Job drawing, mm, ordinate dimensions from the low corner. One solid piece. Give positions to 0.01 mm unless a question says otherwise; leave off trailing zeros. Loops run counter-clockwise (first coordinate to the right, second up) from the corner with the lowest first, then second, coordinate; pieces in that order, holes last.
Item 1: Saw through at C-C on z = 19. Give the cut face in (x, y).
Item 2: Saw through at A-A on z = 39.5. Give the cut face in (x, y) (1 decimal).
Item 3: Saw through at B-B on x = 20.5. Give the cut face in (y, z).
Item 4: Probe probe 1 along Z at (x, y) = (47, 1.85); probe 2 along X at (y, z) = (1.5, 20.5). List the from-to ranges inside material, lowest first.
Item 5: Drop flat-ended pins along their axis: P1, Ø0.9, axis at y = 2, z = 1, coming from the +X side (1 decimal); P2, Ø0.9, axis at y = 1.5, z = 36, coming from the +X side; P3, Ø0.9, axis at x = 1.5, y = 2, coming from the +Z side. Give the stop position or say it passes through.
Item 6: Saw through at D-D on y = 2.2. Give the number of separate pieces and of enclosed holes in the cut face, plus the area to 3 significant figures.
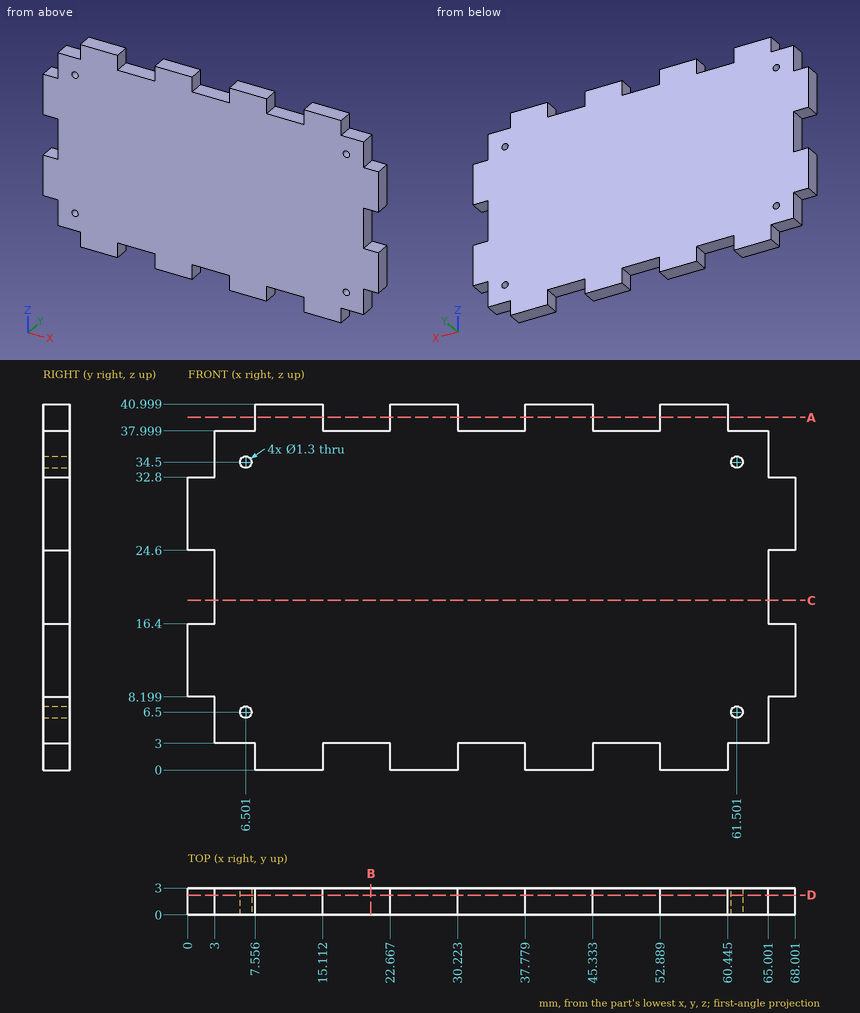
Results below:
1. outline: (3, 0) - (65, 0) - (65, 3) - (3, 3) - close
2. outline: (7.6, 0) - (15.1, 0) - (15.1, 3) - (7.6, 3) - close; (22.7, 0) - (30.2, 0) - (30.2, 3) - (22.7, 3) - close; (37.8, 0) - (45.3, 0) - (45.3, 3) - (37.8, 3) - close; (52.9, 0) - (60.4, 0) - (60.4, 3) - (52.9, 3) - close
3. outline: (0, 3) - (3, 3) - (3, 38) - (0, 38) - close
4. probe 1: z = 3 to 38
4. probe 2: x = 3 to 65
5. P1: stops at x = 60.4
5. P2: stops at x = 65
5. P3: stops at z = 32.8
6. separate pieces: 1
6. enclosed holes: 4
6. area: 2,440 mm2
